Work out the finished part from the listing and answer in its coordinate system (mm). A direction names the side the tool comes from. Coordinates: 2 decimals unless noted, no trailing zeros. Order: outer loops, then holes, each group sorted by start corner. A loop starts at its lowest first (then second) coordinate and runs counter-clockwise, first axis right, second up. Notation, with made-up numbers: M -40,13.25 L -33,13.25 A33 cw -33,50.25 Z; hole C 66,71 d2. An arc over 180 degrees is marked long. Use a Markdown table: item, result.
from build123d import *

# Parameters (mm, degrees)
SKETCH_R      = 1.375
SKETCH_W      = 11
SKETCH_H      = 5.5
PAD_DEPTH     = 0.4
SKETCH001_W   = 35.5
SKETCH001_H   = 35.5
PAD001_DEPTH  = 1.45
SKETCH002_R   = 3.25
SKETCH002_R_2 = 1.375
SKETCH002_R_3 = 3
SKETCH002_R_4 = 2.5
PAD002_DEPTH  = 1.45


with BuildPart() as part:
    # Sketch (on DatumPlane) → Pad (new body)
    with BuildSketch(Plane(origin=(300.2309, 104.1, -11.25), x_dir=(-1, 0, 0), z_dir=(0, 0, -1))):
        Polygon((20.325114, -17.125786), (16.896686, -20.554214), (16.3109, -19.14), (-16.5891, -19.14), (-17.174886, -20.554214), (-20.603314, -17.125786), (-19.1891, -16.54), (-19.1891, 16.36), (-20.603314, 16.945786), (-17.174886, 20.374214), (-16.5891, 18.96), (16.3109, 18.96), (16.896686, 20.374214), (20.325114, 16.945786), (18.9109, 16.36), (18.9109, -16.54), align=None)
        with Locations((-14.1391, 13.91)):
            Circle(SKETCH_R, mode=Mode.SUBTRACT)
        with Locations((13.8609, 13.91)):
            Circle(SKETCH_R, mode=Mode.SUBTRACT)
        with Locations((13.8609, -14.09)):
            Circle(SKETCH_R, mode=Mode.SUBTRACT)
        with Locations((-14.1391, -14.09)):
            Circle(SKETCH_R, mode=Mode.SUBTRACT)
        with Locations((5, 13.25)):
            Rectangle(SKETCH_W, SKETCH_H, mode=Mode.SUBTRACT)
    extrude(amount=-PAD_DEPTH)

    # Sketch001 (on DatumPlane) → Pad001 (join)
    with BuildSketch(Plane(origin=(300.2309, 104.1, -10.85), x_dir=(-1, 0, 0), z_dir=(0, 0, 1))):
        Polygon((16.3109, -18.96), (16.896686, -20.374214), (20.325114, -16.945786), (18.9109, -16.36), (18.9109, 16.54), (20.325114, 17.125786), (16.896686, 20.554214), (16.3109, 19.14), (-16.5891, 19.14), (-17.174886, 20.554214), (-20.603314, 17.125786), (-19.1891, 16.54), (-19.1891, -16.36), (-20.603314, -16.945786), (-17.174886, -20.374214), (-16.5891, -18.96), align=None)
        with Locations((-0.1391, 0.09)):
            Rectangle(SKETCH001_W, SKETCH001_H, mode=Mode.SUBTRACT)
    extrude(amount=PAD001_DEPTH)

    # Sketch002 (on DatumPlane) → Pad002 (join)
    with BuildSketch(Plane(origin=(300.2309, 104.1, -10.85), x_dir=(-1, 0, 0), z_dir=(0, 0, 1))):
        with Locations((-14.1391, -13.91)):
            Circle(SKETCH002_R)
        with Locations((-14.1391, -13.91)):
            Circle(SKETCH002_R_2, mode=Mode.SUBTRACT)
        with Locations((13.8609, 14.09)):
            Circle(SKETCH002_R_3)
        with Locations((13.8609, 14.09)):
            Circle(SKETCH002_R_2, mode=Mode.SUBTRACT)
        with Locations((13.8609, -13.91)):
            Circle(SKETCH002_R)
        with Locations((13.8609, -13.91)):
            Circle(SKETCH002_R_2, mode=Mode.SUBTRACT)
        Circle(SKETCH002_R_4)
        with BuildLine():
            ThreePointArc((-12.5391, 16.918869), (-17.3891, 14.09), (-12.5391, 11.261131))
            Line((-12.5391, 11.261131), (-12.5391, 16.918869))
        make_face()
        with Locations((-14.1391, 14.09)):
            Circle(SKETCH002_R_2, mode=Mode.SUBTRACT)
    extrude(amount=PAD002_DEPTH)


solid = part.part
(1) Determine the mould class of faces 5 (the flat face through (282.62, 104, -10)), 6 (the flat face through (320.12, 120.75, -10.34)), 7 (the flat face through (283.62, 84.24, -10.34)), 8 (the flat face through (316, 90, -9.4)) for opening direction Y: pulls with the +Y half, pulls with the -Y half, needs draft (parallel to the pull), parting line crosses it, or undercut.
Conclusion:
| item | result |
|---|---|
| face 5 | undercut |
| face 6 | undercut |
| face 7 | pulls with the -Y half |
| face 8 | needs draft |
(2) A cutting plane is placed at A-A (z = -9.75). Give the number of separate pieces and of enclosed holes in the cut face, then the cut area to 3 significant figures.
Conclusion:
| item | result |
|---|---|
| separate pieces | 6 |
| enclosed holes | 5 |
| area | 319 mm2 |
(3) Which of the six approach directions +Z, -Z, +X, -X, +Y, -Y give full straight-line access (tool end or side, diameter ignored) to faces 1 (the flat face through (319.42, 104, -10)), 2 (the flat face through (317.12, 123.78, -10.34)), 3 (the flat face through (280.6, 120.76, -10.34)), 4 (the cylindrical face through (302.215, 105.621, -10.135))?
Conclusion:
| item | result |
|---|---|
| face 1 | +Z, -Z, +X |
| face 2 | +Z, -Z, +Y |
| face 3 | +Z, -Z, -X |
| face 4 | +Z |
(4) Straight lines are drawn through the part: L1, parallel to Y at x = 314.37, z = -11 (3 decimals); L2, parallel to X at y = 90.01, z = -9.8 (3 decimals); L3, parallel to X at y = 118.01, z = -10.4 (3 decimals). For each, find the intervals that lie inside material, in ascending order.
Conclusion:
| item | result |
|---|---|
| L1 | 84.96 to 88.635, 91.385 to 116.635, 119.385 to 123.06 |
| L2 | 281.32 to 282.62, 283.37 to 284.995, 287.745 to 289.37, 312.77 to 312.995, 315.745 to 317.62, 318.12 to 319.42 |
| L3 | 281.32 to 282.62, 283.12 to 284.995, 287.745 to 289.62, 311.12 to 312.995, 315.745 to 317.62, 318.12 to 319.42 |
(5) A cutting plane is placed at B-B (x = 314.37). Determine the outline of the cut face in (y, z) (3 decimals).
Conclusion:
| item | result |
|---|---|
| outline | M 84.96,-11.25 L 88.635,-11.25 L 88.635,-9.4 L 86.76,-9.4 L 86.76,-10.85 L 86.26,-10.85 L 86.26,-9.4 L 84.96,-9.4 Z; M 91.385,-11.25 L 116.635,-11.25 L 116.635,-9.4 L 114.76,-9.4 L 114.76,-10.85 L 93.26,-10.85 L 93.26,-9.4 L 91.385,-9.4 Z; M 119.385,-11.25 L 123.06,-11.25 L 123.06,-9.4 L 121.76,-9.4 L 121.76,-10.85 L 121.26,-10.85 L 121.26,-9.4 L 119.385,-9.4 Z |
(6) A cutting plane is placed at D-D (y = 118.01). Determine the outline of the cut face in (x, z) (3 decimals).
Conclusion:
| item | result |
|---|---|
| outline | M 281.32,-11.25 L 284.995,-11.25 L 284.995,-9.4 L 283.12,-9.4 L 283.12,-10.85 L 282.62,-10.85 L 282.62,-9.4 L 281.32,-9.4 Z; M 287.745,-11.25 L 289.731,-11.25 L 289.731,-10.85 L 289.62,-10.85 L 289.62,-9.4 L 287.745,-9.4 Z; M 300.731,-11.25 L 312.995,-11.25 L 312.995,-9.4 L 311.12,-9.4 L 311.12,-10.85 L 300.731,-10.85 Z; M 315.745,-11.25 L 319.42,-11.25 L 319.42,-9.4 L 318.12,-9.4 L 318.12,-10.85 L 317.62,-10.85 L 317.62,-9.4 L 315.745,-9.4 Z |
(7) A cutting plane is placed at C-C (y = 90.01). Determine the outline of the cut face in (x, z) (3 decimals).
Conclusion:
| item | result |
|---|---|
| outline | M 281.32,-11.25 L 284.995,-11.25 L 284.995,-9.4 L 283.37,-9.4 L 283.37,-10.85 L 282.62,-10.85 L 282.62,-9.4 L 281.32,-9.4 Z; M 287.745,-11.25 L 312.995,-11.25 L 312.995,-9.4 L 312.77,-9.4 L 312.77,-10.85 L 289.37,-10.85 L 289.37,-9.4 L 287.745,-9.4 Z; M 315.745,-11.25 L 319.42,-11.25 L 319.42,-9.4 L 318.12,-9.4 L 318.12,-10.85 L 317.62,-10.85 L 317.62,-9.4 L 315.745,-9.4 Z |
(8) Given P1, Ø4, axis at x = 310, y = 90, coming from the +Z side; P2, Ø2, axis at x = 314.37, y = 90.01, coming from the -Z side; P3, Ø0.9, axis at y = 112, z = -10.5, coming from the -X side; P4, Ø10, axis at x = 312.5, y = 94, coming from the +Z side, each flat-ended and moving along its own axis, determine where each tip first touches the part or whether it passes through.
Conclusion:
| item | result |
|---|---|
| P1 | z = -10.85 |
| P2 | through |
| P3 | x = 281.32 |
| P4 | z = -9.4 |
